The listing builds one solid part. Answer for the finished solid, in the listing's coordinates (mm). A direction names the side the tool comes from. Coordinates: 2 decimals unless noted, no trailing zeros. Loops run counter-clockwise (first coordinate to the right, second up) from the corner with the lowest first, then second, coordinate; pieces in that order, holes last. Notation, with made-up numbers: (75, 85) -> (115, 85) arc R23 cw to (115, 109) -> close; hole circle Ø3 at (-14.75, -37). An arc over 180 degrees is marked (long way). Answer in a Markdown table with one row per item.
```python
from build123d import *

# Parameters (mm, degrees)
SKETCH1_W           = 12
SKETCH1_H           = 25.2
BOSS_EXTRUDE1_DEPTH = 3
FILLET1_R           = 6
SKETCH3_W           = 12
SKETCH3_H           = 20
BOSS_EXTRUDE2_DEPTH = 1
FILLET2_R           = 6
CUT_EXTRUDE1_DEPTH  = 3
SKETCH5_R           = 2.8
CUT_EXTRUDE2_DEPTH  = 126.573231257
SKETCH6_R           = 1
CUT_EXTRUDE3_DEPTH  = 126.573231257


with BuildPart() as part:
    # Sketch1 → Boss-Extrude1 (new body)
    with BuildSketch(Plane.XY.offset(5)):
        with Locations((-54.027704131, 97.655662644)):
            Rectangle(SKETCH1_W, SKETCH1_H)
    extrude(amount=BOSS_EXTRUDE1_DEPTH)

    # Fillet1
    fillet1_edges = [part.edges().sort_by_distance(p)[0] for p in [
        (-48.027704131, 85.055662644, 6.5),
        (-60.027704131, 85.055662644, 6.5),
    ]]
    fillet(fillet1_edges, radius=FILLET1_R - 0.0001)  # a hair under: the kernel refuses the full size

    # Sketch3 → Boss-Extrude2 (add)
    with BuildSketch(Plane.XY.offset(8)):
        with Locations((-54.027704131, 95.017998247)):
            Rectangle(SKETCH3_W, SKETCH3_H)
    extrude(amount=BOSS_EXTRUDE2_DEPTH)

    # Fillet2
    fillet2_edges = [part.edges().sort_by_distance(p)[0] for p in [
        (-48.027704131, 85.017998247, 8.5),
        (-60.027704131, 85.017998247, 8.5),
    ]]
    fillet(fillet2_edges, radius=FILLET2_R - 0.0001)  # a hair under: the kernel refuses the full size

    # Sketch4 → Cut-Extrude1 (cut, symmetric)
    with BuildSketch(Plane.XY.offset(9)):
        with BuildLine():
            Line((-56.13842392, 104.48600769), (-51.86157608, 104.48600769))
            Line((-51.86157608, 104.48600769), (-50.824897766, 90.586959839))
            ThreePointArc((-50.824897766, 90.586959839), (-54.164460237, 87.789583498), (-57.199226379, 90.914993286))
            Line((-57.199226379, 90.914993286), (-56.13842392, 104.48600769))
        make_face()
    extrude(amount=CUT_EXTRUDE1_DEPTH, both=True, mode=Mode.SUBTRACT)

    # Sketch5 → Cut-Extrude2 (cut, through all)
    with BuildSketch(Plane.XY.offset(6)):
        with Locations((-53.997448325, 91.08203191)):
            Circle(SKETCH5_R)
    extrude(amount=-CUT_EXTRUDE2_DEPTH, mode=Mode.SUBTRACT)

    # Sketch6 → Cut-Extrude3 (cut, through all)
    with BuildSketch(Plane.XY.offset(8)):
        with Locations((-57.999885247, 107.886757068)):
            Circle(SKETCH6_R)
        with Locations((-49.934118523, 107.886757068)):
            Circle(SKETCH6_R)
    extrude(amount=-CUT_EXTRUDE3_DEPTH, mode=Mode.SUBTRACT)


solid = part.part
```
Item 1: A tool of negligible diameter and unlimited length cuts with its end or side. For faces 4 (the face through (-58.317, 86.86, 6.521)), 5 (the face through (-54, 104.486, 8)), 6 (the face through (-54, 110.256, 6)), 7 (the face through (-54.1, 105.018, 8.5)), 8 (the face through (-54, 98, 5)), from which of +Z, -Z, +X, -X, +Y, -Y can it reach the whole face along a straight path? Write none if from no direction.
Findings below:
| item | result |
|---|---|
| face 4 | -Z, -X, -Y |
| face 5 | +Z |
| face 6 | +Z, -Z, +X, -X, +Y |
| face 7 | +Z, +X, -X, +Y |
| face 8 | -Z, +X, -X, +Y, -Y |
Item 2: Find the intervals of material crossed by probe 1 along X at (y, z) = (108, 6.2); probe 2 along Z at (x, y) = (-57.25, 106); probe 3 along X at (y, z) = (92, 6.25), in increasing order.
Findings below:
| item | result |
|---|---|
| probe 1 | x = -60.03 to -58.99, -57.01 to -50.93, -48.94 to -48.03 |
| probe 2 | z = 5 to 8 |
| probe 3 | x = -60.03 to -57.11, -50.93 to -48.03 |
Item 3: Flat-ended cylindrical pins translate along their axes: pin 1 Ø2 at (y, z) = (88.5, 8.5) entering from -X; pin 2 Ø0.5 at (x, z) = (-55.5, 8.5) entering from +Y; pin 3 Ø1.9 at (x, y) = (-53, 97.5) entering from +Z. Find the tip coordinate at first contact, or state that the pin passes through.
Findings below:
| item | result |
|---|---|
| pin 1 | stops at x = -59.83 |
| pin 2 | stops at y = 105.02 |
| pin 3 | stops at z = 6 |
Item 4: Determine the mould class of faces 1 (the face through (-49.8, 86.8, 6.5)), 2 (the face through (-54, 108, 8)), 3 (the face through (-54.604, 88.349, 5.507)) for opening direction Y: +Y half, -Y half, draft (parallel to the pull), parting line (faces both ways), or undercut.
Findings below:
| item | result |
|---|---|
| face 1 | -Y half |
| face 2 | draft |
| face 3 | undercut |
Item 5: A cutting plane is placed at D-D, the plane y = 108.5. Determine the outline of the cut face in (x, z), plus the area to 3 significant figures.
Findings below:
| item | result |
|---|---|
| outline | (-60.03, 5) -> (-58.79, 5) -> (-58.79, 8) -> (-60.03, 8) -> close; (-57.21, 5) -> (-50.72, 5) -> (-50.72, 8) -> (-57.21, 8) -> close; (-49.14, 5) -> (-48.03, 5) -> (-48.03, 8) -> (-49.14, 8) -> close |
| area | 26.5 mm2 |
Item 6: A cutting plane is placed at C-C, the plane z = 6.9. Count the separate pieces of the cut face and the enclosed holes in it, plus the area to 3 significant figures.
Findings below:
| item | result |
|---|---|
| separate pieces | 1 |
| enclosed holes | 3 |
| area | 193 mm2 |
